Autodesk Inventor part; units mm, degrees
ref_plane "YZ Plane" through (0, 0, 0) normal (1, 0, 0) x (0, 1, 0)
ref_plane "XZ Plane" through (0, 0, 0) normal (0, 1, 0) x (-1, 0, 0)
ref_plane "XY Plane" through (0, 0, 0) normal (0, 0, 1) x (1, 0, 0)
sketch "スケッチ1" plane through (0, 0, 0) normal (0, 0, 1) x (1, 0, 0)
  line L0 (-26.4547, 10.8836) -> (-2.4547, 10.8836)
  line L1 (-2.4547, 10.8836) -> (-2.4547, -14.1164)
  line L2 (-2.4547, -14.1164) -> (-26.4547, -14.1164)
  line L3 (-26.4547, -14.1164) -> (-26.4547, 10.8836)
  point P0 (0, 0)
  dimension "d0" = 25
  dimension "d1" = 24
extrude "押し出し1" add sketch "スケッチ1" along normal blind 15
sketch "スケッチ3" plane through (0, 0, 0) normal (0, 0, -1) x (-1, 0, 0)
  circle A0 centre (10.4547, -3.5864) radius 5
  line L0 (26.4547, 10.8836) -> (2.4547, 10.8836)
  line L1 (2.4547, 10.8836) -> (2.4547, -14.1164)
  point P0 (0, 0)
  dimension "d7" = 10
  dimension "d8" = 14.47
  dimension "d9" = 8
extrude "押し出し2" cut sketch "スケッチ3" against normal blind 10
fillet "フィレット1" radius 5 8 edges at (-2.4547, -14.1164, 7.5) (-14.4547, -14.1164, 15) (-14.4547, -14.1164, 0) (-26.4547, -1.6164, 15) (-26.4547, -14.1164, 7.5) (-26.4547, -1.6164, 0) (-2.4547, -1.6164, 15) (-2.4547, -1.6164, 0)
sketch "スケッチ4" plane through (-21.4547, 10.8836, 0) normal (0, 1, 0) x (1, 0, 0)
  arc A0 (19, -5) -> (14, 0) centre (14, -5) ccw
  line L0 (0, 0) -> (14, 0)
  arc A1 (0, 0) -> (-5, -5) centre (0, -5) ccw
  line L1 (-5, -5) -> (-5, -10)
  arc A2 (-5, -10) -> (0, -15) centre (0, -10) ccw
  line L2 (14, -15) -> (0, -15)
  arc A3 (14, -15) -> (19, -10) centre (14, -10) ccw
  line L3 (19, -5) -> (19, -10)
  circle A4 centre (14.5, -7.5) radius 1.65
  circle A5 centre (-0.5, -7.5) radius 1.65
  point P0 (21.4547, 0)
  dimension "d13" = 3.3
  dimension "d14" = 4.5
  dimension "d15" = 7.5
  dimension "d22" = 15
  dimension "d23" = 3.3
  dimension "d24" = 7.5
extrude "押し出し3" cut sketch "スケッチ4" against normal blind 7 contours A4 | A5
properties part number "door_parts" material "PAEK 樹脂"
Here's how the part is built. I have some questions about the finished solid (model axes, mm). A direction names the side the tool comes from. Coordinates: 2 decimals unless noted, no trailing zeros. Write each loop counter-clockwise with the first axis right and the second up, starting at its lowest first coordinate (ties: lowest second). Pieces come first, ordered by that corner, then holes.
Item 1: On a 3-axis mill with a long thin cutter (end or side, diameter ignored), from which of +Z, -Z, +X, -X, +Y, -Y can I reach the whole of each face in a straight line? I mean faces 4 (the flat face through (-7, 3.884, 7)), 5 (the flat face through (-14, -14.116, 7)), 6 (the cylindrical face through (-15.224, -2.085, 4.93)). Say none if no direction works.
Item 2: I want a section at C-C on x = -10.5. Write out the boundary of the cut face in (y, z).
Item 3: Will these pins go through, and if not, where does the flat tip stop? pin 1 (9 mm diameter, centred on x = -10.45, y = -3.59, fed in from -Z); pin 2 (2 mm diameter, centred on y = -10.5, z = 2, fed in from -X); pin 3 (1 mm diameter, centred on x = -22, z = 8, fed in from +Y).
Item 4: If I drill on line 1 (X direction, y = 8.5, z = 7.5); line 2 (Y direction, x = -6.25, z = 5.5); line 3 (Y direction, x = -11.75, z = 2), over which ranges is the centre line in solid material (lowest first)?
Item 5: I want a section at D-D on y = 0. Write out the boundary of the cut face in (x, z).
Item 6: I want a section at A-A on y = 8.75. Write out the boundary of the cut face in (x, z).
Item 7: If we mould it in two halves opening along Y, with no side actions, what happens to faces 1 (the cylindrical face through (-24.95, -12.69, 7.46)), 2 (the cylindrical face through (-8.264, 7.433, 8.504)), 3 (the flat face through (-10, -4, 10))? For each: +Y half, -Y half, draft (parallel to the pull), parting line (faces both ways), or undercut.
Item 8: I want a section at B-B on z = 3.25. Write out the boundary of the cut face in (x, y), and give its area (3 significant figures).
Findings below:
1. face 4: +Y
1. face 5: +Z, -Z, +X, -X, -Y
1. face 6: -Z
2. outline: (-14.12, 5) arc R5 ccw to (-9.12, 0) - (-8.59, 0) - (-8.59, 10) - (1.41, 10) - (1.41, 0) - (10.88, 0) - (10.88, 15) - (-9.12, 15) arc R5 ccw to (-14.12, 10) - close
3. pin 1: stops at z = 10
3. pin 2: stops at x = -25.89
3. pin 3: stops at y = 3.88
4. line 1: x = -26.45 to -23.6, -20.3 to -8.6, -5.3 to -2.45
4. line 2: y = -13.97 to -6.29, -0.88 to 10.88
4. line 3: y = -13.12 to -8.42, 1.24 to 10.88
5. outline: (-26.45, 5) arc R5 ccw to (-21.45, 0) - (-13.94, 0) - (-13.94, 10) - (-6.97, 10) - (-6.97, 0.02) arc R5 ccw to (-2.45, 5) - (-2.45, 10) arc R5 ccw to (-7.45, 15) - (-21.45, 15) arc R5 ccw to (-26.45, 10) - close
6. outline: (-26.45, 5) arc R5 ccw to (-21.45, 0) - (-7.45, 0) arc R5 ccw to (-2.45, 5) - (-2.45, 10) arc R5 ccw to (-7.45, 15) - (-21.45, 15) arc R5 ccw to (-26.45, 10) - close; hole circle Ø3.3 at (-21.95, 7.5); hole circle Ø3.3 at (-6.95, 7.5)
7. face 1: -Y half
7. face 2: draft
7. face 3: undercut
8. outline: (-26.14, -9.12) arc R4.68 ccw to (-21.45, -13.8) - (-7.45, -13.8) arc R4.68 ccw to (-2.77, -9.12) - (-2.77, 10.88) - (-26.14, 10.88) - close; hole circle Ø10 at (-10.45, -3.59)
8. area: 489 mm2
